Design review of the part built by this model. Coordinates are the model's own, in mm. Give positions to 0.01 mm unless a question says otherwise; leave off trailing zeros. Order: outer loops, then holes, each group sorted by start corner. A loop starts at its lowest first (then second) coordinate and runs counter-clockwise, first axis right, second up.
Autodesk Inventor part; units mm, degrees
ref_plane "YZ Plane" through (0, 0, 0) normal (1, 0, 0) x (0, 1, 0)
ref_plane "XZ Plane" through (0, 0, 0) normal (0, 1, 0) x (-1, 0, 0)
ref_plane "XY Plane" through (0, 0, 0) normal (0, 0, 1) x (1, 0, 0)
sketch "Sketch1" plane through (0, 0, 0) normal (0, 1, 0) x (-1, 0, 0)
  line L0 (58.3565, 287.7551) -> (-176.5935, 287.7551)
  line L1 (-176.5935, -271.0449) -> (58.3565, -271.0449)
  line L2 (58.3565, -271.0449) -> (58.3565, 287.7551)
  line L3 (-176.5935, 287.7551) -> (-176.5935, 135.3551)
  line L4 (-176.5935, 135.3551) -> (-328.9935, 135.3551)
  line L5 (-328.9935, -118.6449) -> (-176.5935, -118.6449)
  line L6 (-176.5935, -118.6449) -> (-176.5935, -271.0449)
  line L7 (-328.9935, 135.3551) -> (-328.9935, 76.6176)
  line L8 (-328.9935, -59.9074) -> (-328.9935, -118.6449)
  line L9 (-328.9935, -59.9074) -> (-328.9935, 76.6176)
  dimension "d3" = 558.8
  dimension "d4" = 234.95
  dimension "d5" = 152.4
  dimension "d6" = 152.4
  dimension "d11" = 152.4
  dimension "d12" = 234.95
extrude "Plate1" add sketch "Sketch1" along normal blind 4.7625
equation "\"BendRadius\" = Thickness"
equation "\"BendReliefWidth\" = Thickness"
equation "\"BendReliefDepth\" = 0.5 * Thickness"
equation "\"CornerReliefSize\" = 4 * Thickness"
equation "\"MinimumRemnant\" = 2 * Thickness"
equation "\"TransitionRadius\" = BendRadius"
equation "\"JacobiRadiusSize\" = BendRadius"
equation "\"GapSize\" = Thickness"
equation "\"d9\" = BendRadius"
properties part number "top_bottom_rev2" material "Steel, Mild"
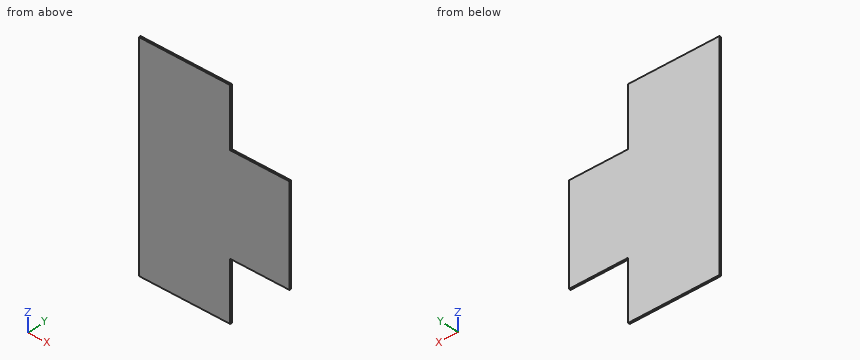
1. Take a section at A-A (y = 3.75). State the section outline as (x, z) points, then the cut area to 3 significant figures.
Recorded:
outline: (-58.36, -271.04) - (176.59, -271.04) - (176.59, -118.64) - (328.99, -118.64) - (328.99, 135.36) - (176.59, 135.36) - (176.59, 287.76) - (-58.36, 287.76) - close
area: 170,000 mm2
2. For line 1 along X through (y, z) = (3.35, -236); line 2 along Z through (x, y) = (195.5, 2.9), list the stretches that pass through material, from the lowest coordinate up.
Recorded:
line 1: x = -58.36 to 176.59
line 2: z = -118.64 to 135.36
3. Take a section at B-B (z = -166.5). State the section outline as (x, y) points.
Recorded:
outline: (-58.36, 0) - (176.59, 0) - (176.59, 4.76) - (-58.36, 4.76) - close
4. Take a section at C-C (x = 190). State the section outline as (y, z) points, then the cut area to 3 significant figures.
Recorded:
outline: (0, -118.64) - (4.76, -118.64) - (4.76, 135.36) - (0, 135.36) - close
area: 1,210 mm2
5. For pin 1 (2 mm diameter, centred on x = 275, y = 4, fed in from -Z); pin 2 (10 mm diameter, centred on x = 180.5, z = -192.5, fed in from +Y); pin 3 (1.4 mm diameter, centred on y = 3, z = -165, fed in from +X), all flat-tipped, find the tip position at first contact; note any pin that passes through.
Recorded:
pin 1: stops at z = -118.64
pin 2: stops at y = 4.76
pin 3: stops at x = 176.59
